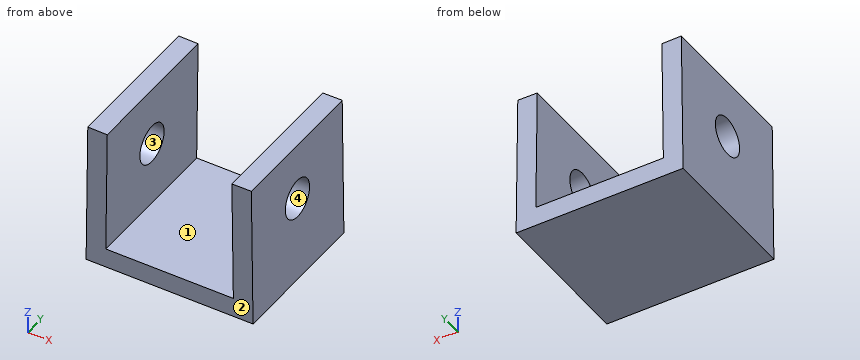
```python
from build123d import *

# Parameters (mm, degrees)
BOSS_EXTRUDE1_DEPTH      = 30
SKETCH3_R                = 4
CUT_EXTRUDE1_DEPTH       = 40
SKETCH4_W                = 3
SKETCH4_H                = 41
BOSS_EXTRUDE2_DEPTH      = 4
BOSS_EXTRUDE3_DEPTH      = 25
BOSS_EXTRUDE3_DEPTH_BACK = 4
SKETCH5_W                = 3
SKETCH5_H                = 7.75
BOSS_EXTRUDE4_REACH      = 69.734
SKETCH6_W                = 4
SKETCH6_H                = 56.5
CUT_EXTRUDE2_DEPTH       = 62


with BuildPart() as part:
    # Sketch1 → Boss-Extrude1 (new body)
    with BuildSketch(Plane(origin=(0, 0, 0), x_dir=(1, 0, 0), z_dir=(0, 1, 0))):
        Polygon((-12.8, -12.8), (-13.1, 12.8), (13.1, 12.8), (12.8, -12.6), (16.799721029, -12.6472408), (17.147523085, 16.8), (-17.147149649, 16.8), (-16.79972537, -12.846871782), align=None)
    extrude(amount=BOSS_EXTRUDE1_DEPTH)

    # Sketch3 → Cut-Extrude1 (cut)
    with BuildSketch(Plane(origin=(16.946733814, 0, 0.200158273), x_dir=(0.011810199887684227, 0, -0.9999302571572745), z_dir=(0.9999302571572745, 0, 0.011810199887684227))):
        with Locations(Location((-0.747950682, 15, 0), (0, 0, 180))):
            Circle(SKETCH3_R)
    extrude(amount=-CUT_EXTRUDE1_DEPTH, mode=Mode.SUBTRACT)

    # Sketch4 → Boss-Extrude2 (add)
    with BuildSketch(Plane(origin=(0, 0, -16.8), x_dir=(-1, 0, 0), z_dir=(0, 0, -1))):
        with Locations((12.499813282, 15)):
            Rectangle(SKETCH4_W, SKETCH4_H)
    extrude(amount=-BOSS_EXTRUDE2_DEPTH)

    # Sketch5 → Boss-Extrude3 (add, two sides: drawn at the far end of the back side and taken through both)
    with BuildSketch(Plane(origin=(0, 0, -16.8), x_dir=(-1, 0, 0), z_dir=(0, 0, -1)).offset(-BOSS_EXTRUDE3_DEPTH_BACK)):
        with Locations((12.499813282, 39.375)):
            Rectangle(SKETCH5_W, SKETCH5_H)
        with Locations((12.499813282, -9.375)):
            Rectangle(SKETCH5_W, SKETCH5_H)
    extrude(amount=BOSS_EXTRUDE3_DEPTH + BOSS_EXTRUDE3_DEPTH_BACK)

    # Boss-Extrude4: up to this plane
    boss_extrude4_end = Plane(origin=(-16.79972537, 30, 12.846871782), z_dir=(0.9999313425206403, 0, -0.01171794542016394))
    # Sketch6 → Boss-Extrude4 (add, up to the surface)
    with BuildSketch(Plane.ZY.offset(13.999813282), mode=Mode.PRIVATE) as boss_extrude4_sk1:
        with Locations((-14.8, 15)):
            Rectangle(SKETCH6_W, SKETCH6_H)
    boss_extrude4_tool1 = split(extrude(boss_extrude4_sk1.sketch, amount=BOSS_EXTRUDE4_REACH, mode=Mode.PRIVATE), bisect_by=boss_extrude4_end, keep=Keep.BOTH, mode=Mode.PRIVATE)
    add(boss_extrude4_tool1.solids().sort_by_distance((-13.999813, 15, -14.8))[0])

    # Sketch7 → Cut-Extrude2 (cut)
    with BuildSketch(Plane(origin=(-16.947947202, 0, 0.198608756), x_dir=(0.01171794542016394, 0, 0.9999313425206403), z_dir=(-0.9999313425206403, 0, 0.01171794542016394))):
        Polygon((12.649131483, 30), (-40.255802642, 30), (-53.566220107, 38.891145172), (-52.192714639, 50.02792354), (-13.80333558, 48.779139174), (23.506142402, 46.053591691), (14.671560105, 30), align=None)
        Polygon((12.649131483, 0), (-49.960950266, 0), (-43.210741963, -24.331655391), (11.653429031, -25.806337238), (35.291011187, -15.934393486), (29.689158759, -2.52120452), align=None)
    extrude(amount=-CUT_EXTRUDE2_DEPTH, mode=Mode.SUBTRACT)


solid = part.part
```
Part model, mm, in its own coordinate system. Face numbers are marked on the shaded views. Round coordinates to 2 decimals unless told otherwise and drop trailing zeros. Loops run counter-clockwise (first coordinate to the right, second up) from the corner with the lowest first, then second, coordinate; pieces in that order, holes last.
1. Slice it at B-B (z = -10.5). Give the cut face in (x, y), and give its area (3 significant figures).
Solutions:
outline: (-17.07, 0) - (-13.07, 0) - (-13.07, 30) - (-17.07, 30) - close; (13.07, 0) - (17.07, 0) - (17.07, 30) - (13.07, 30) - close
area: 240 mm2
2. Slice it at D-D (x = 0). Give the cut face in (y, z), and give its area (3 significant figures).
Solutions:
outline: (0, -16.8) - (30, -16.8) - (30, -12.8) - (0, -12.8) - close
area: 120 mm2
3. Slice it at A-A (y = 7). Give the cut face in (x, z), and give its area (3 significant figures).
Solutions:
outline: (-17.15, -16.8) - (17.15, -16.8) - (16.8, 12.65) - (12.8, 12.6) - (13.1, -12.8) - (-13.1, -12.8) - (-12.8, 12.8) - (-16.8, 12.85) - close
area: 341 mm2
4. Two-plate mould, pull along Y, no slides. Class the marked faces 1, 2, 3 and 4: pulls with the +Y half, pulls with the -Y half, needs draft (parallel to the pull), parting line crosses it, or undercut.
Solutions:
face 1: needs draft
face 2: pulls with the -Y half
face 3: undercut
face 4: undercut
5. Slice it at C-C (y = 13.25). Give the cut face in (x, z), and give its area (3 significant figures).
Solutions:
outline: (-17.15, -16.8) - (17.15, -16.8) - (16.98, -2.65) - (12.98, -2.7) - (13.1, -12.8) - (-13.1, -12.8) - (-12.99, -3) - (-16.99, -3.05) - close; (-16.9, 4.15) - (-12.9, 4.19) - (-12.8, 12.8) - (-16.8, 12.85) - close; (12.8, 12.6) - (12.9, 4.5) - (16.9, 4.54) - (16.8, 12.65) - close
area: 284 mm2
6. Flat gauge pins, fed straight in: pin 1 (10 mm diameter, centred on y = 12.5, z = -1.5, fed in from -X); pin 2 (8 mm diameter, centred on x = -9, y = 7, fed in from +Z); pin 3 (12 mm diameter, centred on x = 13, y = 23, fed in from +Z). Where does each tip first touch, or does it go through?
Solutions:
pin 1: stops at x = -17.03
pin 2: stops at z = 12.8
pin 3: stops at z = 12.65
7. Drill centre lines: line 1 along Z through (x, y) = (8.5, 24.5); line 2 along X through (y, z) = (5, 0.5); line 3 along X through (y, z) = (21, -9.5). Where is each one in solid material? Low to high.
Solutions:
line 1: z = -16.8 to -12.8
line 2: x = -16.94 to -12.94, 12.94 to 16.94
line 3: x = -17.06 to -13.06, 13.06 to 17.06
